```python
from build123d import *

# Parameters (mm, degrees)
SK_P01_BUMPERFACE_W      = 5
SK_P01_BUMPERFACE_H      = 13
P01_BUMPERFACE_DEPTH     = 43
SK_P02_BUMPERFACE_W      = 5
SK_P02_BUMPERFACE_H      = 59
P02_BUMPERFACE_DEPTH     = 43
SK_P03_BUMPERFACE_W      = 5
SK_P03_BUMPERFACE_H      = 18
P03_BUMPERFACE_DEPTH     = 10
P04_BUMPERFACE_START     = 34
SK_P04_BUMPERFACE_W      = 5
SK_P04_BUMPERFACE_H      = 18
P04_BUMPERFACE_DEPTH     = 9
P05_FLEXUREBRACKET_START = 31
SK_P05_FLEXUREBRACKET_W  = 30
SK_P05_FLEXUREBRACKET_H  = 12
P05_FLEXUREBRACKET_DEPTH = 6
P06_SWITCHSS5GL2_START   = 20
SK_P06_SWITCHSS5GL2_W    = 6.5
SK_P06_SWITCHSS5GL2_H    = 20
P06_SWITCHSS5GL2_DEPTH   = 10.2
SK_P07_BUMPERFACE_W      = 5
SK_P07_BUMPERFACE_H      = 13
P07_BUMPERFACE_DEPTH     = 43
SK_P08_BUMPERFACE_W      = 5
SK_P08_BUMPERFACE_H      = 59
P08_BUMPERFACE_DEPTH     = 43
SK_P09_BUMPERFACE_W      = 5
SK_P09_BUMPERFACE_H      = 18
P09_BUMPERFACE_DEPTH     = 10
P10_BUMPERFACE_START     = 34
SK_P10_BUMPERFACE_W      = 5
SK_P10_BUMPERFACE_H      = 18
P10_BUMPERFACE_DEPTH     = 9
P11_FLEXUREBRACKET_START = 31
SK_P11_FLEXUREBRACKET_W  = 30
SK_P11_FLEXUREBRACKET_H  = 12
P11_FLEXUREBRACKET_DEPTH = 6
P12_SWITCHSS5GL2_START   = 20
SK_P12_SWITCHSS5GL2_W    = 6.5
SK_P12_SWITCHSS5GL2_H    = 20
P12_SWITCHSS5GL2_DEPTH   = 10.2
P13_BUMPERFACE_START     = 26
SK_P13_BUMPERFACE_W      = 5
SK_P13_BUMPERFACE_H      = 70
P13_BUMPERFACE_DEPTH     = 17


with BuildPart() as part:
    # SK_P01_Bumperface → P01_Bumperface (new body)
    with BuildSketch(Plane(origin=(0, 0, 0), x_dir=(1, 0, 0), z_dir=(0, 1, 0))):
        with Locations((15, -41.5)):
            Rectangle(SK_P01_BUMPERFACE_W, SK_P01_BUMPERFACE_H)
    extrude(amount=P01_BUMPERFACE_DEPTH)



with BuildPart() as body_2:
    # SK_P02_Bumperface → P02_Bumperface (new body)
    with BuildSketch(Plane(origin=(0, 0, 0), x_dir=(1, 0, 0), z_dir=(0, 1, 0))):
        with Locations((15, -95.5)):
            Rectangle(SK_P02_BUMPERFACE_W, SK_P02_BUMPERFACE_H)
    extrude(amount=P02_BUMPERFACE_DEPTH)


with BuildPart() as part_1:
    add(part.part)

    add(body_2.part)  # P03_Bumperface merges body 2
    # SK_P03_Bumperface → P03_Bumperface (add)
    with BuildSketch(Plane(origin=(0, 0, 0), x_dir=(1, 0, 0), z_dir=(0, 1, 0))):
        with Locations((15, -57)):
            Rectangle(SK_P03_BUMPERFACE_W, SK_P03_BUMPERFACE_H)
    extrude(amount=P03_BUMPERFACE_DEPTH)

    # SK_P04_Bumperface → P04_Bumperface (add)
    with BuildSketch(Plane(origin=(0, 0, 0), x_dir=(1, 0, 0), z_dir=(0, 1, 0)).offset(P04_BUMPERFACE_START)):
        with Locations((15, -57)):
            Rectangle(SK_P04_BUMPERFACE_W, SK_P04_BUMPERFACE_H)
    extrude(amount=P04_BUMPERFACE_DEPTH)

    # SK_P05_Flexurebracket → P05_Flexurebracket (add)
    with BuildSketch(Plane(origin=(0, 0, 0), x_dir=(1, 0, 0), z_dir=(0, 1, 0)).offset(P05_FLEXUREBRACKET_START)):
        with Locations((-2.5, -112)):
            Rectangle(SK_P05_FLEXUREBRACKET_W, SK_P05_FLEXUREBRACKET_H)
    extrude(amount=P05_FLEXUREBRACKET_DEPTH)

    # SK_P06_SwitchSS5GL2 → P06_SwitchSS5GL2 (add)
    with BuildSketch(Plane(origin=(0, 0, 0), x_dir=(1, 0, 0), z_dir=(0, 1, 0)).offset(P06_SWITCHSS5GL2_START)):
        with Locations((9.25, -98)):
            Rectangle(SK_P06_SWITCHSS5GL2_W, SK_P06_SWITCHSS5GL2_H)
    extrude(amount=P06_SWITCHSS5GL2_DEPTH)



with BuildPart() as body_2_2:
    # SK_P07_Bumperface → P07_Bumperface (new body)
    with BuildSketch(Plane(origin=(0, 0, 0), x_dir=(1, 0, 0), z_dir=(0, 1, 0))):
        with Locations((15, 41.5)):
            Rectangle(SK_P07_BUMPERFACE_W, SK_P07_BUMPERFACE_H)
    extrude(amount=P07_BUMPERFACE_DEPTH)



with BuildPart() as body_3:
    # SK_P08_Bumperface → P08_Bumperface (new body)
    with BuildSketch(Plane(origin=(0, 0, 0), x_dir=(1, 0, 0), z_dir=(0, 1, 0))):
        with Locations((15, 95.5)):
            Rectangle(SK_P08_BUMPERFACE_W, SK_P08_BUMPERFACE_H)
    extrude(amount=P08_BUMPERFACE_DEPTH)


with BuildPart() as body_2_2_1:
    add(body_2_2.part)

    add(body_3.part)  # P09_Bumperface merges body 3
    # SK_P09_Bumperface → P09_Bumperface (add)
    with BuildSketch(Plane(origin=(0, 0, 0), x_dir=(1, 0, 0), z_dir=(0, 1, 0))):
        with Locations((15, 57)):
            Rectangle(SK_P09_BUMPERFACE_W, SK_P09_BUMPERFACE_H)
    extrude(amount=P09_BUMPERFACE_DEPTH)

    # SK_P10_Bumperface → P10_Bumperface (add)
    with BuildSketch(Plane(origin=(0, 0, 0), x_dir=(1, 0, 0), z_dir=(0, 1, 0)).offset(P10_BUMPERFACE_START)):
        with Locations((15, 57)):
            Rectangle(SK_P10_BUMPERFACE_W, SK_P10_BUMPERFACE_H)
    extrude(amount=P10_BUMPERFACE_DEPTH)

    # SK_P11_Flexurebracket → P11_Flexurebracket (add)
    with BuildSketch(Plane(origin=(0, 0, 0), x_dir=(1, 0, 0), z_dir=(0, 1, 0)).offset(P11_FLEXUREBRACKET_START)):
        with Locations((-2.5, 112)):
            Rectangle(SK_P11_FLEXUREBRACKET_W, SK_P11_FLEXUREBRACKET_H)
    extrude(amount=P11_FLEXUREBRACKET_DEPTH)

    # SK_P12_SwitchSS5GL2 → P12_SwitchSS5GL2 (add)
    with BuildSketch(Plane(origin=(0, 0, 0), x_dir=(1, 0, 0), z_dir=(0, 1, 0)).offset(P12_SWITCHSS5GL2_START)):
        with Locations((9.25, 98)):
            Rectangle(SK_P12_SWITCHSS5GL2_W, SK_P12_SWITCHSS5GL2_H)
    extrude(amount=P12_SWITCHSS5GL2_DEPTH)


with BuildPart() as part_2:
    add(part_1.part)

    add(body_2_2_1.part)  # P13_Bumperface merges body 2 2
    # SK_P13_Bumperface → P13_Bumperface (add)
    with BuildSketch(Plane(origin=(0, 0, 0), x_dir=(1, 0, 0), z_dir=(0, 1, 0)).offset(P13_BUMPERFACE_START)):
        with Locations((15, 0)):
            Rectangle(SK_P13_BUMPERFACE_W, SK_P13_BUMPERFACE_H)
    extrude(amount=P13_BUMPERFACE_DEPTH)


solid = part_2.part
```
Work out the finished part from the listing and answer in its coordinate system (mm). A direction names the side the tool comes from. Give positions to 0.01 mm unless a question says otherwise; leave off trailing zeros. Order: outer loops, then holes, each group sorted by start corner. A loop starts at its lowest first (then second) coordinate and runs counter-clockwise, first axis right, second up. Notation, with made-up numbers: M -38,81 L -32,81 A17 ccw -32,95 Z; hole C 47.25,28.25 d6. An arc over 180 degrees is marked long. Return JSON: item names as keys, results as strings.
1) Section A-A, the plane x = 9 is taken. Write down the section's boundary in (y, z), plus the area to 3 significant figures.
Resolved:
{"outline": "M 20,-108 L 30.2,-108 L 30.2,-88 L 20,-88 Z; M 20,88 L 30.2,88 L 30.2,108 L 20,108 Z; M 31,-118 L 37,-118 L 37,-106 L 31,-106 Z; M 31,106 L 37,106 L 37,118 L 31,118 Z", "area": "552 mm^2"}
2) Section C-C, the plane y = 15.5 is taken. Write down the section's boundary in (x, z), plus the area to 3 significant figures.
Resolved:
{"outline": "M 12.5,-125 L 17.5,-125 L 17.5,-66 L 12.5,-66 Z; M 12.5,-48 L 17.5,-48 L 17.5,-35 L 12.5,-35 Z; M 12.5,35 L 17.5,35 L 17.5,48 L 12.5,48 Z; M 12.5,66 L 17.5,66 L 17.5,125 L 12.5,125 Z", "area": "720 mm^2"}
3) For a pull along Z with two mould halves and no side action, classify faces 5 (the flat face through (15, 10, -57)), 6 (the flat face through (-17.5, 34, -112)), 7 (the flat face through (-3, 34, 118)) as +Z half, -Z half, draft (parallel to the pull), parting line (faces both ways), or undercut.
Resolved:
{"face 5": "undercut", "face 6": "draft", "face 7": "+Z half"}
4) Section D-D, the plane x = -5 is taken. Write down the section's boundary in (y, z).
Resolved:
{"outline": "M 31,-118 L 37,-118 L 37,-106 L 31,-106 Z; M 31,106 L 37,106 L 37,118 L 31,118 Z"}
5) Straight lines are drawn through the part: line 1 along Y through (x, z) = (7, -90); line 2 along Z through (x, y) = (10, 29); line 3 along X through (y, z) = (11, 37.5). For each, find the intervals that lie inside material, in ascending order. Write a range as [from, to].
Resolved:
{"line 1": "[20, 30.2]", "line 2": "[-108, -88], [88, 108]", "line 3": "[12.5, 17.5]"}
6) A tool of negligible diameter and unlimited length cuts with its end or side. For faces 1 (the flat face through (9, 25, 108)), 2 (the flat face through (15, 34, -57)), 3 (the flat face through (9, 25, -108)), 4 (the flat face through (9, 20, -98)), from which of +Z, -Z, +X, -X, +Y, -Y can it reach the whole face along a straight path? Write none if from no direction.
Resolved:
{"face 1": "+Z, -X, -Y", "face 2": "+X, -X", "face 3": "-Z, -X, -Y", "face 4": "+Z, -Z, -X, -Y"}
7) Each of these flat-tipped pins is pushed along its axis until it touches: pin 1 (3 mm diameter, centred on x = 8.5, z = -96, fed in from +Y); pin 2 (13 mm diameter, centred on x = 1, z = -109.5, fed in from -Y); pin 3 (2 mm diameter, centred on x = 9, y = 26, fed in from -Z); pin 4 (3 mm diameter, centred on x = 12.5, z = -83.5, fed in from -Y). Where does it stop, or does it pass through?
Resolved:
{"pin 1": "y = 30.2", "pin 2": "y = 20", "pin 3": "z = -108", "pin 4": "y = 0"}
8) Section B-B, the plane z = 60 is taken. Write down the section's boundary in (x, y), plus the area to 3 significant figures.
Resolved:
{"outline": "M 12.5,0 L 17.5,0 L 17.5,10 L 12.5,10 Z; M 12.5,34 L 17.5,34 L 17.5,43 L 12.5,43 Z", "area": "95.0 mm^2"}
